Work out the finished part from the listing and answer in its coordinate system (mm). A direction names the side the tool comes from. Round coordinates to 2 decimals unless told otherwise and drop trailing zeros. Write each loop counter-clockwise with the first axis right and the second up, starting at its lowest first coordinate (ties: lowest second). Pieces come first, ordered by that corner, then holes.
1. Straight lines are drawn through the part: probe 1 along Z at (x, y) = (7.5, 2.45); probe 2 along Z at (x, y) = (6.5, 5.2); probe 3 along X at (y, z) = (3.05, 7). For each, find the intervals that lie inside material, in ascending order.
2. Find section B-B (y = 3.1). Write down the section's boundary in (x, z), and give its area (3 significant figures).
3. Flat-ended cylindrical pins translate along their axes: pin 1 Ø1.5 at (y, z) = (3, 9) entering from -X; pin 2 Ø1.2 at (y, z) = (3, 6.5) entering from +X; pin 3 Ø2.5 at (x, y) = (9.5, 3) entering from +Z. Find the tip coordinate at first contact, or state that the pin passes through.
4. Find section D-D (z = 3). Write down the section's boundary in (x, y), and give its area (3 significant figures).
5. Find section A-A (x = 10). Write down the section's boundary in (y, z).
6. A tool of negligible diameter and unlimited length cuts with its end or side. For faces 1 (the face through (0, 2, 7)), 2 (the face through (10, 2, 0)), 3 (the face through (20, 2, 7)), 4 (the face through (10, 3, 5.75)), 5 (the face through (10, 2, 14)), from which of +Z, -Z, +X, -X, +Y, -Y can it reach the whole face along a straight path? Write none if from no direction.
7. Find section C-C (z = 7.5). Write down the section's boundary in (x, y).
8. Determine the mould class of faces 6 (the face through (15, 3, 7)), 7 (the face through (10, 6, 9)), 8 (the face through (-1, 5.5, 7.1)) for opening direction X: pulls with the +X half, pulls with the -X half, needs draft (parallel to the pull), parting line crosses it, or undercut.
```python
from build123d import *

# Parameters (mm, degrees)
SKETCH1_W           = 20
SKETCH1_H           = 14
SKETCH1_W_2         = 10
SKETCH1_H_2         = 2.5
BOSS_EXTRUDE1_DEPTH = 5
SKETCH2_W           = 22
SKETCH2_H           = 16
SKETCH2_W_2         = 10
SKETCH2_H_2         = 2.5
BOSS_EXTRUDE2_DEPTH = 1
FILLET1_R           = 0.5


with BuildPart() as part:
    # Sketch1 → Boss-Extrude1 (new body)
    with BuildSketch(Plane(origin=(0, 0, 0), x_dir=(1, 0, 0), z_dir=(0, 1, 0))):
        with Locations((10, -7)):
            Rectangle(SKETCH1_W, SKETCH1_H)
        with Locations((10, -7)):
            Rectangle(SKETCH1_W_2, SKETCH1_H_2, mode=Mode.SUBTRACT)
    extrude(amount=BOSS_EXTRUDE1_DEPTH)

    # Sketch2 → Boss-Extrude2 (add)
    with BuildSketch(Plane(origin=(0, 5, 0), x_dir=(1, 0, 0), z_dir=(0, 1, 0))):
        with Locations((10, -7)):
            Rectangle(SKETCH2_W, SKETCH2_H)
        with Locations((10, -7)):
            Rectangle(SKETCH2_W_2, SKETCH2_H_2, mode=Mode.SUBTRACT)
    extrude(amount=BOSS_EXTRUDE2_DEPTH)

    # Fillet1
    fillet1_edges = [part.edges().sort_by_distance(p)[0] for p in [
        (15, 3, 8.25),
        (15, 3, 5.75),
        (5, 3, 5.75),
        (5, 3, 8.25),
        (0, 2.5, 0),
        (20, 2.5, 0),
        (20, 2.5, 14),
        (0, 2.5, 14),
    ]]
    fillet(fillet1_edges, radius=FILLET1_R)


solid = part.part
```
Worked answers:
1. probe 1: z = 0 to 5.75, 8.25 to 14
1. probe 2: z = -1 to 5.75, 8.25 to 15
1. probe 3: x = 0 to 5, 15 to 20
2. outline: (0, 0.5) arc R0.5 ccw to (0.5, 0) - (19.5, 0) arc R0.5 ccw to (20, 0.5) - (20, 13.5) arc R0.5 ccw to (19.5, 14) - (0.5, 14) arc R0.5 ccw to (0, 13.5) - close; hole (5, 6.25) arc R0.5 ccw to (5.5, 5.75) - (14.5, 5.75) arc R0.5 ccw to (15, 6.25) - (15, 7.75) arc R0.5 ccw to (14.5, 8.25) - (5.5, 8.25) arc R0.5 ccw to (5, 7.75) - close
2. area: 255 mm2
3. pin 1: stops at x = 0
3. pin 2: stops at x = 20
3. pin 3: stops at z = 14
4. outline: (-1, 5) - (0, 5) - (0, 0) - (20, 0) - (20, 5) - (21, 5) - (21, 6) - (-1, 6) - close
4. area: 122 mm2
5. outline: (0, 0) - (5, 0) - (5, -1) - (6, -1) - (6, 5.75) - (0, 5.75) - close; (0, 8.25) - (6, 8.25) - (6, 15) - (5, 15) - (5, 14) - (0, 14) - close
6. face 1: +Z, -Z, -X, -Y
6. face 2: -Z, +X, -X, -Y
6. face 3: +Z, -Z, +X, -Y
6. face 4: +Y, -Y
6. face 5: +Z, +X, -X, -Y
7. outline: (-1, 5) - (0, 5) - (0, 0) - (5, 0) - (5, 6) - (-1, 6) - close; (15, 0) - (20, 0) - (20, 5) - (21, 5) - (21, 6) - (15, 6) - close
8. face 6: undercut
8. face 7: needs draft
8. face 8: pulls with the -X half
